For this review, take the finished solid that the model builds, in its own axes (mm). A direction names the side the tool comes from. Round coordinates to 2 decimals unless told otherwise and drop trailing zeros. Order: outer loops, then holes, each group sorted by start corner. A loop starts at its lowest first (then second) coordinate and runs counter-clockwise, first axis right, second up. Notation, with made-up numbers: M 48,25.5 L 106,25.5 A23 ccw 106,38.5 Z; hole C -38,10.5 d8. An arc over 180 degrees is marked long. Use a Markdown table: item, result.
from build123d import *

# Parameters (mm, degrees)
F0_W      = 570
F0_H      = 32
F1_DEPTH  = 13
F3_DEPTH  = 570
F4_W      = 3
F4_H      = 18
F5_DEPTH  = 8
F6_W      = 8
F6_H      = 3
F7_DEPTH  = 102
F8_W      = 3
F8_H      = 15
F9_DEPTH  = 12
F10_W     = 3
F10_H     = 102
F10_H_2   = 18
F11_DEPTH = 8
F12_W     = 3
F12_H     = 15
F13_DEPTH = 12


with BuildPart() as f1:
    # F0 (on Top) → F1 (new body)
    with BuildSketch(Plane.XY):
        Rectangle(F0_W, F0_H)
    extrude(amount=F1_DEPTH)

    # F2 (on face) → F3 (join)
    with BuildSketch(Plane(origin=(-285, 0, 0), x_dir=(0, -1, 0), z_dir=(-1, 0, 0))):
        Polygon((-16, 13), (16, 13), (28, 35), (-16, 35), align=None)
    extrude(amount=-F3_DEPTH)

    # F4 (on face) → F5 (join)
    with BuildSketch(Plane(origin=(-285, 0, 0), x_dir=(0, -1, 0), z_dir=(-1, 0, 0))):
        with Locations((0, 26)):
            Rectangle(F4_W, F4_H)
    extrude(amount=F5_DEPTH)

    # F6 (on face) → F7 (join)
    with BuildSketch(Plane.XY.offset(35)):
        with Locations((-289, 0)):
            Rectangle(F6_W, F6_H)
    extrude(amount=F7_DEPTH)

    # F8 (on face) → F9 (join)
    with BuildSketch(Plane.YZ.offset(-285)):
        with Locations((0, 129.5)):
            Rectangle(F8_W, F8_H)
    extrude(amount=F9_DEPTH)

    # F10 (on face) → F11 (join)
    with BuildSketch(Plane.YZ.offset(285)):
        with Locations((0, 86)):
            Rectangle(F10_W, F10_H)
        with Locations((0, 26)):
            Rectangle(F10_W, F10_H_2)
    extrude(amount=F11_DEPTH)

    # F12 (on face) → F13 (join)
    with BuildSketch(Plane(origin=(285, 0, 0), x_dir=(0, -1, 0), z_dir=(-1, 0, 0))):
        with Locations((0, 129.5)):
            Rectangle(F12_W, F12_H)
    extrude(amount=F13_DEPTH)


solid = f1.part
Q1. Add section C-C (z = 128). Write out the cut boundary in (x, y), then the cut area to 3 significant figures.
Determined:
| item | result |
|---|---|
| outline | M -293,-1.5 L -273,-1.5 L -273,1.5 L -293,1.5 Z; M 273,-1.5 L 293,-1.5 L 293,1.5 L 273,1.5 Z |
| area | 120 mm^2 |
Q2. Machinability: for faces 1 (the flat face through (-4, 0, 0)), 2 (the flat face through (-4, -16, 6)), which of the approach directions +Z, -Z, +X, -X, +Y, -Y give a long, thin tool a straight path to every point of the face, cutting with its end or side? Answer none if there is none.
Determined:
| item | result |
|---|---|
| face 1 | -Z, +X, -X, +Y, -Y |
| face 2 | -Z, +X, -X, -Y |
Q3. Add section A-A (z = 94). Write out the cut boundary in (x, y), then the cut area to 3 significant figures.
Determined:
| item | result |
|---|---|
| outline | M -293,-1.5 L -285,-1.5 L -285,1.5 L -293,1.5 Z; M 285,-1.5 L 293,-1.5 L 293,1.5 L 285,1.5 Z |
| area | 48.0 mm^2 |
Q4. Wall thickness on line 1 along X through (y, z) = (1, 65); line 2 along Z through (x, y) = (97, 7); line 3 along X through (y, z) = (10, 31.5): over which ranges is each line inside the solid? List them lowest first. Write a range as [from, to].
Determined:
| item | result |
|---|---|
| line 1 | x = [-293, -285], [285, 293] |
| line 2 | z = [0, 35] |
| line 3 | x = [-285, 285] |
Q5. Add section B-B (x = -160.5). Write out the cut boundary in (y, z).
Determined:
| item | result |
|---|---|
| outline | M -28,35 L -16,13 L -16,0 L 16,0 L 16,35 Z |
Q6. Add section D-D (z = 27). Write out the cut boundary in (x, y), then the cut area to 3 significant figures.
Determined:
| item | result |
|---|---|
| outline | M -293,-1.5 L -285,-1.5 L -285,-23.64 L 285,-23.64 L 285,-1.5 L 293,-1.5 L 293,1.5 L 285,1.5 L 285,16 L -285,16 L -285,1.5 L -293,1.5 Z |
| area | 22,600 mm^2 |
Q7. Clearance check with flat-ended pins moving along their axes: pin 1 (6 mm diameter, centred on x = -285, z = 93.5, fed in from -Y); pin 2 (6 mm diameter, centred on x = -284.5, z = 60, fed in from +Y); pin 3 (0.9 mm diameter, centred on x = -287.5, y = -0.5, fed in from -Z). State where each tip first meets the part, or that it passes through.
Determined:
| item | result |
|---|---|
| pin 1 | stops at y = -1.5 |
| pin 2 | stops at y = 1.5 |
| pin 3 | stops at z = 17 |
